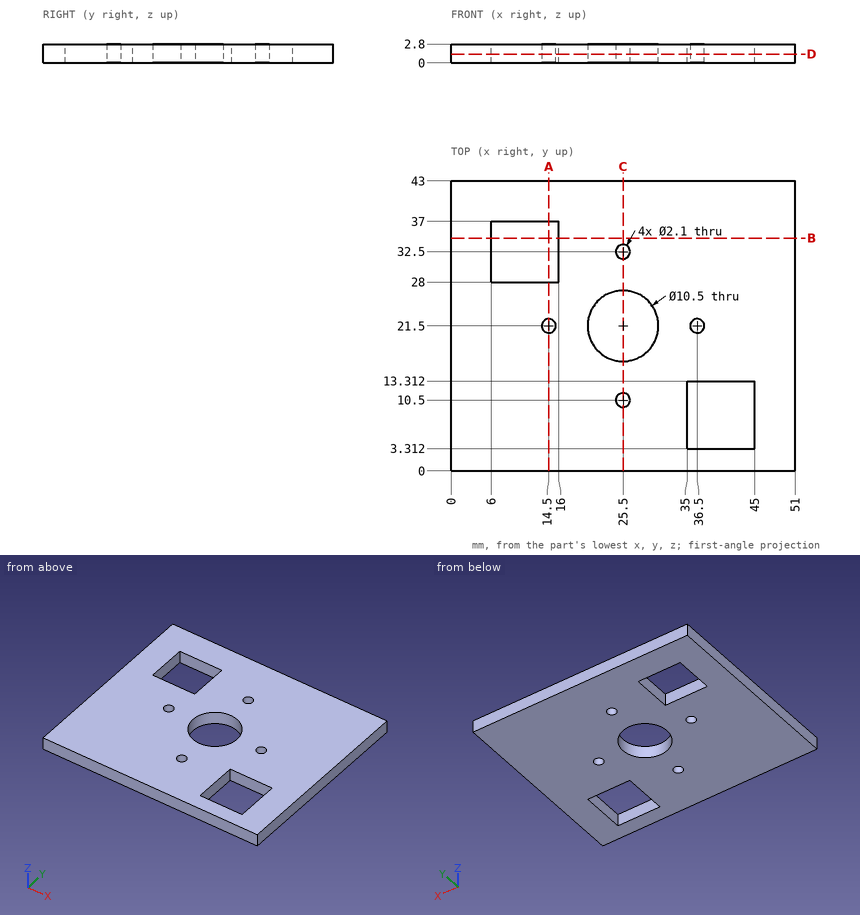
Part print with two shaded views. Sizes in mm from the minimum x, y, z corner. Round coordinates to 2 decimals unless told otherwise and drop trailing zeros. Order: outer loops, then holes, each group sorted by start corner. A loop starts at its lowest first (then second) coordinate and runs counter-clockwise, first axis right, second up. Notation, with made-up numbers: M 23.5,50 L 43.5,50 A21 ccw 43.5,55 Z; hole C 8,36 d9. An arc over 180 degrees is marked long. Answer in a Markdown table with one row per item. Add a question column.
Q1. Pin check, flat tip, straight feed: pin 1 (1.3 mm diameter, centred on x = 25.5, y = 32.5, fed in from +Z). Stop position of the tip, or through.
Q2. Wall check: L1, parallel to X at y = 32.5, z = 1.85; L2, parallel to Y at x = 25.5, z = 1.85; L3, parallel to X at y = 35, z = 1.4. Give the ranges that are in metal, low to high. Write a range as from..to.
Q3. Cut at D-D on z = 1.3. Give the cut face in (x, y).
Q4. Cut at A-A on x = 14.5. Give the cut face in (y, z).
Q5. Cut at B-B on y = 34.5. Give the cut face in (x, z).
Q6. Cut at C-C on x = 25.5. Give the cut face in (y, z).
Established:
| question | item | result |
|---|---|---|
| 1 | pin 1 | passes through |
| 2 | L1 | x = 0..6, 16..24.45, 26.55..51 |
| 2 | L2 | y = 0..9.45, 11.55..16.25, 26.75..31.45, 33.55..43 |
| 2 | L3 | x = 0..6, 16..51 |
| 3 | outline | M 0,0 L 51,0 L 51,43 L 0,43 Z; hole M 6,28 L 16,28 L 16,37 L 6,37 Z; hole C 14.5,21.5 d2.1; hole C 25.5,21.5 d10.5; hole C 25.5,10.5 d2.1; hole C 25.5,32.5 d2.1; hole M 35,3.31 L 45,3.31 L 45,13.31 L 35,13.31 Z; hole C 36.5,21.5 d2.1 |
| 4 | outline | M 0,0 L 20.45,0 L 20.45,2.8 L 0,2.8 Z; M 22.55,0 L 28,0 L 28,2.8 L 22.55,2.8 Z; M 37,0 L 43,0 L 43,2.8 L 37,2.8 Z |
| 5 | outline | M 0,0 L 6,0 L 6,2.8 L 0,2.8 Z; M 16,0 L 51,0 L 51,2.8 L 16,2.8 Z |
| 6 | outline | M 0,0 L 9.45,0 L 9.45,2.8 L 0,2.8 Z; M 11.55,0 L 16.25,0 L 16.25,2.8 L 11.55,2.8 Z; M 26.75,0 L 31.45,0 L 31.45,2.8 L 26.75,2.8 Z; M 33.55,0 L 43,0 L 43,2.8 L 33.55,2.8 Z |
